from build123d import *

# Parameters (mm, degrees)
F0_R     = 1.5
F0_R_2   = 1.55
F1_DEPTH = 8
F3_DEPTH = 3
F4_R     = 1.55
F5_DEPTH = 8.001
F6_R     = 3.05
F7_DEPTH = 4
F8_R     = 5


with BuildPart() as f1:
    # F0 (on Front) → F1 (new body)
    with BuildSketch(Plane.XZ):
        Polygon((55, -6), (55, 18.586979), (0, 25.823821), (-32.46, 25.823821), (-32.46, 18.123821), (-32.46, 10.423821), (-11.26, 10.423821), (0, 0), (0, -6), align=None)
        with Locations((5, 0)):
            Circle(F0_R, mode=Mode.SUBTRACT)
        with Locations((48, 0)):
            Circle(F0_R, mode=Mode.SUBTRACT)
        Polygon((10, 5), (9.393527, 14.28), (44.444109, 9.668081), (43, 5), align=None, mode=Mode.SUBTRACT)
        with Locations((-27.46, 18.123821)):
            Circle(F0_R_2, mode=Mode.SUBTRACT)
        with Locations((-16.26, 18.123821)):
            Circle(F0_R_2, mode=Mode.SUBTRACT)
        with Locations((3.74, 19.28)):
            Circle(F0_R, mode=Mode.SUBTRACT)
        with Locations((52, 12.93)):
            Circle(F0_R, mode=Mode.SUBTRACT)
    extrude(amount=F1_DEPTH)

    # F2 (on face) → F3 (cut)
    with BuildSketch(Plane(origin=(0, 0, 0), x_dir=(-1, 0, 0), z_dir=(0, 1, 0))):
        Polygon((-49, 11.197949), (-49, 14.662051), (-52, 16.394102), (-55, 14.662051), (-55, 11.197949), (-52, 9.465898), align=None)
        Polygon((-45, -1.732051), (-45, 1.732051), (-48, 3.464102), (-51, 1.732051), (-51, -1.732051), (-48, -3.464102), align=None)
        Polygon((-8, 1.732051), (-8, -1.732051), (-5, -3.464102), (-2, -1.732051), (-2, 1.732051), (-5, 3.464102), align=None)
        Polygon((-6.74, 21.012051), (-6.74, 17.547949), (-3.74, 15.815898), (-0.74, 17.547949), (-0.74, 21.012051), (-3.74, 22.744102), align=None)
    extrude(amount=-F3_DEPTH, mode=Mode.SUBTRACT)

    # F4 (on face) → F5 (cut, through all)
    with BuildSketch(Plane.XZ.offset(8)):
        with Locations((16.5, 0)):
            Circle(F4_R)
        with Locations((36.5, 0)):
            Circle(F4_R)
        with Locations((16.5, 17.601053)):
            Circle(F4_R)
        with Locations((36.5, 14.969474)):
            Circle(F4_R)
    extrude(amount=-F5_DEPTH, mode=Mode.SUBTRACT)

    # F6 (on face) → F7 (cut)
    with BuildSketch(Plane.XZ.offset(8)):
        with Locations((16.5, 0)):
            Circle(F6_R)
        with Locations((36.5, 0)):
            Circle(F6_R)
        with Locations((16.5, 17.601053)):
            Circle(F6_R)
        with Locations((36.5, 14.969474)):
            Circle(F6_R)
    extrude(amount=-F7_DEPTH, mode=Mode.SUBTRACT)

    # F8
    f8_edges = [f1.edges().sort_by_distance(p)[0] for p in [
        (-32.46, -4, 25.823821),
        (-32.46, -4, 10.423821),
        (-11.26, -4, 10.423821),
        (0, -4, -6),
        (55, -4, -6),
        (55, -4, 18.586979),
    ]]
    fillet(f8_edges, radius=F8_R)


solid = f1.part
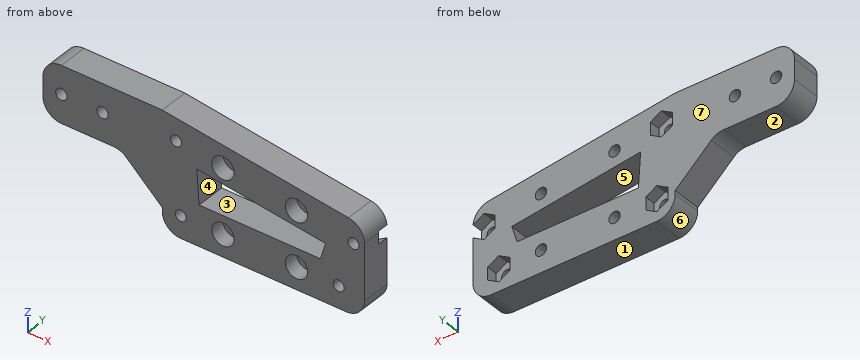
Verification items for the finished model (mm, model axes). Face numbers are marked on the shaded views. A direction names the side the tool comes from. Round coordinates to 2 decimals unless told otherwise and drop trailing zeros. Loops run counter-clockwise (first coordinate to the right, second up) from the corner with the lowest first, then second, coordinate; pieces in that order, holes last. Notation, with made-up numbers: (61, 3) - (90, 3) arc R24 ccw to (90, 42) - close; hole circle Ø11 at (37.25, 7). An arc over 180 degrees is marked (long way). Use a Markdown table: item, result. Add a question column.
1. Thickness scan on probe 1 along X at (y, z) = (-5.5, 2.5); probe 2 along Z at (x, y) = (16.5, -1.35); probe 3 along X at (y, z) = (-6, 18.5). Record the ranges inside material, lowest first. Write a range as [from, to].
2. Section check D-D, the plane x = 29. Record the boundary of the cut face in (y, z).
3. Section check C-C, the plane y = -6. Give the number of separate pieces and of enclosed holes in the cut face, plus the area to 3 significant figures.
4. Release check for a two-part mould opening along Z. For the marked faces 4, 5, 6 and 7 record: released by +Z, released by -Z, zero draft, split by the parting line, or undercut.
5. Gauge pin test, flat ends, axial feed: pin 1 (1.5 mm diameter, centred on y = -1, z = 0.5, fed in from -X); pin 2 (0.8 mm diameter, centred on y = -4.5, z = -0.5, fed in from -X); pin 3 (1 mm diameter, centred on y = -5, z = 8, fed in from -X); pin 4 (3 mm diameter, centred on x = 16.5, z = 17.6, fed in from +Y). Record the tip position at first contact, or that the pin passes through.
6. Section check A-A, the plane x = 16.5. Record the boundary of the cut face in (y, z), plus the area to 3 significant figures.
7. Section check B-B, the plane z = 6.5. Record the boundary of the cut face in (x, y).
8. Access from +Z, -Z, +X, -X, +Y, -Y to the whole of each face (thin tool, end or side, straight path). Record for the marked faces 1, 2 and 3.
Checks:
| question | item | result |
|---|---|---|
| 1 | probe 1 | x = [-2.7, 14.75], [18.25, 34.75], [38.25, 55] |
| 1 | probe 2 | z = [-6, -1.55], [1.55, 5], [13.34, 16.05], [19.15, 23.65] |
| 1 | probe 3 | x = [-32.46, -28.96], [-25.96, -17.76], [-14.76, 2.46], [5.02, 13.59], [19.41, 52.55] |
| 2 | outline | (-8, -6) - (0, -6) - (0, 5) - (-8, 5) - close; (-8, 11.7) - (0, 11.7) - (0, 22.01) - (-8, 22.01) - close |
| 3 | separate pieces | 1 |
| 3 | enclosed holes | 11 |
| 3 | area | 1,690 mm^2 |
| 4 | face 4 | undercut |
| 4 | face 5 | undercut |
| 4 | face 6 | released by -Z |
| 4 | face 7 | zero draft |
| 5 | pin 1 | stops at x = -1.35 |
| 5 | pin 2 | stops at x = 0 |
| 5 | pin 3 | stops at x = -9.18 |
| 5 | pin 4 | passes through |
| 6 | outline | (-8, -6) - (0, -6) - (0, -1.55) - (-4, -1.55) - (-4, -3.05) - (-8, -3.05) - close; (-8, 3.05) - (-4, 3.05) - (-4, 1.55) - (0, 1.55) - (0, 5) - (-8, 5) - close; (-8, 13.34) - (0, 13.34) - (0, 16.05) - (-4, 16.05) - (-4, 14.55) - (-8, 14.55) - close; (-8, 20.65) - (-4, 20.65) - (-4, 19.15) - (0, 19.15) - (0, 23.65) - (-8, 23.65) - close |
| 6 | area | 96.9 mm^2 |
| 7 | outline | (-7.02, -8) - (9.9, -8) - (9.9, 0) - (-7.02, 0) - close; (43.46, -8) - (55, -8) - (55, 0) - (43.46, 0) - close |
| 8 | face 1 | -Z, +X, -X, +Y, -Y |
| 8 | face 2 | -Z, -X, +Y, -Y |
| 8 | face 3 | +Y, -Y |
